Geometry check sheet. Reference: the model listing, model coordinates, mm. Face numbers are marked on the shaded views. A direction names the side the tool comes from. Coordinates: 2 decimals unless noted, no trailing zeros. Write each loop counter-clockwise with the first axis right and the second up, starting at its lowest first coordinate (ties: lowest second). Pieces come first, ordered by that corner, then holes.
Autodesk Inventor part; units mm, degrees
ref_plane "YZ Plane" through (0, 0, 0) normal (1, 0, 0) x (0, 1, 0)
ref_plane "XZ Plane" through (0, 0, 0) normal (0, 1, 0) x (-1, 0, 0)
ref_plane "XY Plane" through (0, 0, 0) normal (0, 0, 1) x (1, 0, 0)
sketch "Sketch1" plane through (0, 0, 0) normal (0, 0, 1) x (1, 0, 0)
  line L0 (-245, 20) -> (245, 20)
  line L1 (245, 20) -> (245, -20)
  line L2 (245, -20) -> (-245, -20)
  line L3 (-245, -20) -> (-245, 20)
  point P0 (0, 0)
  dimension "d0" = 490
  dimension "d1" = 40
  dimension "d2" = 20
  dimension "d3" = 245
extrude "Plate1" add sketch "Sketch1" along normal blind 3
sketch "Sketch2" plane through (0, 0, 3) normal (0, 0, 1) x (1, 0, 0)
  line L0 (-245, 20) -> (245, 20)
  line L1 (-245, -20) -> (-245, 20)
  arc A0 (-232.25, 12.5) -> (-237.75, 12.5) centre (-235, 12.5) ccw
  arc A1 (-237.75, -12.5) -> (-232.25, -12.5) centre (-235, -12.5) ccw
  line L2 (-237.75, 12.5) -> (-237.75, -12.5)
  line L3 (-232.25, -12.5) -> (-232.25, 12.5)
  point P0 (0, 0)
  dimension "d5" = 5.5
  dimension "d6" = 5.5
  dimension "d8" = 10
  dimension "d9" = 10
  dimension "d11" = 7.5
  dimension "d27" = 25
  dimension "d28" = 25
extrude "Extrusion1" cut sketch "Sketch2" against normal blind 10
pattern_linear "Rectangular Pattern1" count 2 spacing 470 along (1, 0, 0) of "Extrusion1"
sketch "Sketch3" plane through (245, 23, -3) normal (0, 1, 0) x (-1, 0, 0)
  line L0 (490, 0) -> (0, 0)
  line L1 (0, 0) -> (0, -19)
  line L2 (0, -19) -> (490, -19)
  line L3 (490, -19) -> (490, 0)
edge flange "Flange1" height 25 angle 90 thickness 3 bend radius 3 thickness toward (0, 1, 0) relief tear relief width 3 relief depth 1.5 edges at (0, 20, 0) wall of the first edge with corners at (-245, 23, -3) (245, 23, -3) (245, 23, -22) (-245, 23, -22)
bend "Bend1"
corner "Corner1"
sketch "Sketch4" plane through (-245, 26, -22) normal (0, 1, 0) x (1, 0, 0)
  line L0 (0, 0) -> (490, 0)
  line L1 (0, -19) -> (0, 0)
  circle A0 centre (10, -9.5) radius 2
  circle A1 centre (110, -9.5) radius 2
  point P0 (245, -22)
  dimension "d29" = 4
  dimension "d30" = 9.5
  dimension "d31" = 10
  dimension "d32" = 4
  dimension "d33" = 110
  dimension "d34" = 9.5
extrude "Extrusion2" cut sketch "Sketch4" against normal through all
pattern_linear "Rectangular Pattern2" count 4 spacing 125 along (1, 0, 0) of "Extrusion2"
sketch "Sketch5" plane through (0, 0, 3) normal (0, 0, 1) x (1, 0, 0)
  line L0 (-245, 20) -> (245, 20)
  line L1 (-245, -20) -> (-245, 20)
  circle A0 centre (-195, 10) radius 2.75
  circle A1 centre (-195, -10) radius 2.75
  point P0 (0, 0)
  dimension "d40" = 5.5
  dimension "d41" = 5.5
  dimension "d42" = 20
  dimension "d43" = 10
  dimension "d44" = 50
  dimension "d45" = 50
extrude "Extrusion3" cut sketch "Sketch5" against normal through all
pattern_linear "Rectangular Pattern3" count 3 spacing 195 along (1, 0, 0) of "Extrusion3"
equation "\"d17\" = BendReliefWidth"
equation "\"d18\" = BendReliefDepth"
equation "\"d19\" = MinimumRemnant"
equation "\"d20\" = BendRadius"
equation "\"d23\" = BendRadius"
equation "\"d24\" = CornerReliefSize"
equation "\"d25\" = GapSize"
equation "\"d26\" = JacobiRadiusSize"
equation "\"BendRadius\" = Thickness"
equation "\"BendReliefWidth\" = Thickness"
equation "\"BendReliefDepth\" = 0.5 * Thickness"
equation "\"CornerReliefSize\" = 4 * Thickness"
equation "\"MinimumRemnant\" = 2 * Thickness"
equation "\"TransitionRadius\" = BendRadius"
equation "\"JacobiRadiusSize\" = BendRadius"
equation "\"GapSize\" = Thickness"
equation "\"d4\" = BendRadius"
properties part number "formed_right_left" material "Steel, Mild"
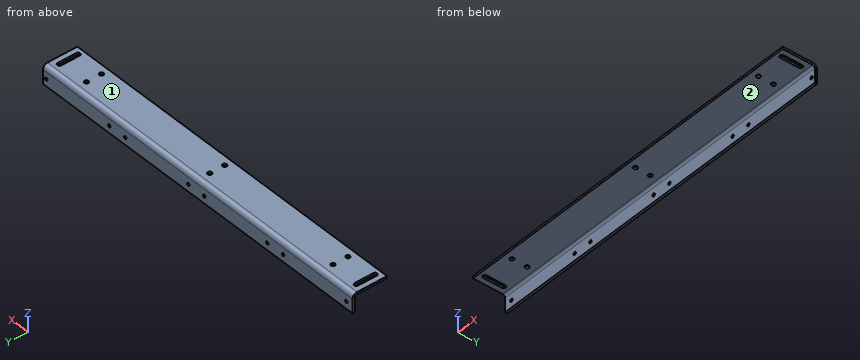
1. Thickness scan on line 1 along X through (y, z) = (-2.5, 0.5); line 2 along Y through (x, z) = (-195, 2.2); line 3 along Y through (x, z) = (0, 1.3). Record the ranges inside material, lowest first.
Computed values:
line 1: x = -245 to -237.75, -232.25 to 232.25, 237.75 to 245
line 2: y = -20 to -12.75, -7.25 to 7.25, 12.75 to 22.99
line 3: y = -20 to -12.75, -7.25 to 7.25, 12.75 to 24.18
2. Sectioned sample at B-B, the plane x = 150.5. Record the boundary of the cut face in (y, z), and give its area (3 significant figures).
Computed values:
outline: (-20, 0) - (20, 0) arc R3 cw to (23, -3) - (23, -22) - (26, -22) - (26, -3) arc R6 ccw to (20, 3) - (-20, 3) - close
area: 198 mm2
3. Sectioned sample at A-A, the plane y = 1. Record the boundary of the cut face in (x, z), and give its area (3 significant figures).
Computed values:
outline: (-245, 0) - (-237.75, 0) - (-237.75, 3) - (-245, 3) - close; (-232.25, 0) - (232.25, 0) - (232.25, 3) - (-232.25, 3) - close; (237.75, 0) - (245, 0) - (245, 3) - (237.75, 3) - close
area: 1,440 mm2
4. Access from +Z, -Z, +X, -X, +Y, -Y to the whole of each face (thin tool, end or side, straight path). Record for the marked faces 1 and 2.
Computed values:
face 1: +Z, +X, -X, +Y, -Y
face 2: -Z, +X, -X, -Y
5. Gauge pin test, flat ends, axial feed: pin 1 Ø4 at (x, z) = (102.5, -1) entering from +Y; pin 2 Ø1.5 at (x, y) = (144.5, 14.5) entering from -Z; pin 3 Ø15 at (x, z) = (8, -16) entering from -Y. Record the tip position at first contact, or that the pin passes through.
Computed values:
pin 1: stops at y = 26
pin 2: stops at z = 0
pin 3: stops at y = 23
